```python
from build123d import *

# Parameters (mm, degrees)
BOSS_EXTRU_1_DEPTH      = 10
ENL_V_MAT_EXTRU_1_DEPTH = 10


with BuildPart() as part:
    # Esquisse1 → Boss.-Extru.1 (new body)
    with BuildSketch(Plane.XY):
        Polygon((-750, 0), (0, 1299.038105677), (750, 0), align=None)
    extrude(amount=BOSS_EXTRU_1_DEPTH)

    # Esquisse2 → Enlèv. mat.-Extru.1 (cut)
    with BuildSketch(Plane.XY.offset(10)):
        Polygon((-746.535898385, 2), (0, 1295.038105677), (746.535898385, 2), align=None)
    extrude(amount=-ENL_V_MAT_EXTRU_1_DEPTH, mode=Mode.SUBTRACT)


solid = part.part
```
Verification items for the finished model (mm, model axes). Coordinates: 2 decimals unless noted, no trailing zeros. Loops run counter-clockwise (first coordinate to the right, second up) from the corner with the lowest first, then second, coordinate; pieces in that order, holes last. Notation, with made-up numbers: (20, 83) -> (66, 83) arc R21 ccw to (66, 115) -> close; hole circle Ø1 at (-7.5, 39). An arc over 180 degrees is marked (long way). Answer in a Markdown table with one row per item. Add a question column.
1. Material ranges on probe 1 along Y at (x, z) = (-187, 9.25); probe 2 along X at (y, z) = (165, 2); probe 3 along Y at (x, z) = (-452, 6.5), recorded low to high. Write a range as [from, to].
2. Section check B-B, the plane y = 140. Enter the section's corners in (x, z).
3. Depth check by flat-ended pin: P1, Ø5, axis at y = 277.5, z = 2, coming from the +X side; P2, Ø2, axis at y = 873, z = 3.5, coming from the +X side; P3, Ø3, axis at x = -535, z = 7, coming from the +Y side. Enter the tip coordinate at first touch or a pass-through.
4. Section check C-C, the plane z = 2.75. Enter the section's corners in (x, y).
5. Section check A-A, the plane x = -651.5. Enter the section's corners in (y, z), then the cut area to 3 significant figures.
6. Draft check along X on faces 1 (the face through (-380.25, 640.426, 4.93)), 2 (the face through (369.75, 658.61, 4.93)), 3 (the face through (368.042, 657.57, 5.07)). Enter one of: +X half, -X half, draft (parallel to the pull), parting line (faces both ways), or undercut.
Derived:
| question | item | result |
|---|---|---|
| 1 | probe 1 | y = [0, 2], [971.14, 975.14] |
| 1 | probe 2 | x = [-654.74, -652.43], [652.43, 654.74] |
| 1 | probe 3 | y = [0, 2], [512.15, 516.15] |
| 2 | outline | (-669.17, 0) -> (-666.86, 0) -> (-666.86, 10) -> (-669.17, 10) -> close; (666.86, 0) -> (669.17, 0) -> (669.17, 10) -> (666.86, 10) -> close |
| 3 | P1 | stops at x = 591.23 |
| 3 | P2 | stops at x = 246.55 |
| 3 | P3 | stops at y = 374.99 |
| 4 | outline | (-750, 0) -> (750, 0) -> (0, 1299.04) -> close; hole (-746.54, 2) -> (746.54, 2) -> (0, 1295.04) -> close |
| 5 | outline | (0, 0) -> (2, 0) -> (2, 10) -> (0, 10) -> close; (166.61, 0) -> (170.61, 0) -> (170.61, 10) -> (166.61, 10) -> close |
| 5 | area | 60.0 mm² |
| 6 | face 1 | -X half |
| 6 | face 2 | +X half |
| 6 | face 3 | undercut |
